The listing builds one solid part. Answer for the finished solid, in the listing's coordinates (mm). A direction names the side the tool comes from. Round coordinates to 2 decimals unless told otherwise and drop trailing zeros. Loops run counter-clockwise (first coordinate to the right, second up) from the corner with the lowest first, then second, coordinate; pieces in that order, holes last. Notation, with made-up numbers: M 23,76.5 L 68,76.5 A15 ccw 68,83.5 Z; hole C 15,87.5 d6. An arc over 180 degrees is marked long. Put each result on its own line as item: value. Start each with the question number.
(1) Section A-A, the plane z = 140 is taken. Determine the outline of the cut face in (x, y), then the cut area to 3 significant figures.
(2) Determine the mould class of faces 5 (the face through (-4.24, 0.751, 137.615)), 6 (the face through (-5, 0, 135)), 7 (the face through (6.466, -2.681, 1.75)) for opening direction Y: released by +Y, released by -Y, zero draft, split by the parting line, or undercut.
(3) Which of the six approach directions +Z, -Z, +X, -X, +Y, -Y give full straight-line access (tool end or side, diameter ignored) to faces 1 (the face through (0, 2, 125)), 2 (the face through (0, 0, -125)), 3 (the face through (5, 0, 135)), 4 (the face through (3.5, 0, 135))?
(4) Flat-ended cylindrical pins translate along their axes: P1, Ø2, axis at y = -4.5, z = 22.5, coming from the -X side; P2, Ø2, axis at y = -0.5, z = 139, coming from the +X side; P3, Ø3.5, axis at y = 0.5, z = 130.5, coming from the -X side; P4, Ø1.2, axis at x = 4.5, z = 136, coming from the -Y side. Find the tip coordinate at first contact, or state that the pin passes through.
(5) Section B-B, the plane z = 19.5 is taken. Determine the outline of the cut face in (x, y).
(6) Straight lines are drawn through the part: line 1 (Z direction, x = 4.3, y = 0); line 2 (Y direction, x = -3.75, z = 140); line 3 (Z direction, x = -0.75, y = 3). For each, find the intervals that lie inside material, in ascending order.
```python
from build123d import *

# Parameters (mm, degrees)
SKETCH1_R                = 7
BOSS_EXTRUDE1_DEPTH      = 125
BOSS_EXTRUDE1_DEPTH_BACK = 125
SKETCH2_W                = 20
SKETCH2_H                = 7
SKETCH2_R                = 2.5
BOSS_EXTRUDE2_DEPTH      = 5
BOSS_EXTRUDE2_DEPTH_BACK = 5
SKETCH4_W                = 7
SKETCH4_H                = 7
CUT_EXTRUDE1_DEPTH       = 20
SKETCH5_R                = 1.5
BOSS_EXTRUDE3_DEPTH      = 5


with BuildPart() as part:
    # Sketch1 → Boss-Extrude1 (new body, two sides)
    with BuildSketch(Plane.XY) as boss_extrude1_sk:
        Circle(SKETCH1_R)
    extrude(amount=BOSS_EXTRUDE1_DEPTH)
    extrude(boss_extrude1_sk.sketch, amount=-BOSS_EXTRUDE1_DEPTH_BACK)

    # Sketch2 → Boss-Extrude2 (add, two sides)
    with BuildSketch(Plane(origin=(0, 0, 0), x_dir=(0, 0, -1), z_dir=(1, 0, 0))) as boss_extrude2_sk:
        with Locations((-135, 0)):
            Rectangle(SKETCH2_W, SKETCH2_H)
        with Locations((-140, 0)):
            Circle(SKETCH2_R, mode=Mode.SUBTRACT)
    extrude(amount=BOSS_EXTRUDE2_DEPTH)
    extrude(boss_extrude2_sk.sketch, amount=-BOSS_EXTRUDE2_DEPTH_BACK)

    # Sketch4 → Cut-Extrude1 (cut)
    with BuildSketch(Plane.XY.offset(145)):
        Rectangle(SKETCH4_W, SKETCH4_H)
    extrude(amount=-CUT_EXTRUDE1_DEPTH, mode=Mode.SUBTRACT)

    # Sketch5 → Boss-Extrude3 (add)
    with BuildSketch(Plane.XY.offset(125)):
        Circle(SKETCH5_R)
    extrude(amount=BOSS_EXTRUDE3_DEPTH)


solid = part.part
```
Recorded:
1. outline: M -5,-3.5 L -3.5,-3.5 L -3.5,-2.5 L -5,-2.5 Z; M -5,2.5 L -3.5,2.5 L -3.5,3.5 L -5,3.5 Z; M 3.5,-3.5 L 5,-3.5 L 5,-2.5 L 3.5,-2.5 Z; M 3.5,2.5 L 5,2.5 L 5,3.5 L 3.5,3.5 Z
1. area: 6.00 mm²
2. face 5: undercut
2. face 6: zero draft
2. face 7: split by the parting line
3. face 1: +Z
3. face 2: -Z, +X, -X, +Y, -Y
3. face 3: +Z, +X, +Y, -Y
3. face 4: +Z, +Y, -Y
4. P1: stops at x = -6.06
4. P2: passes through
4. P3: stops at x = -5
4. P4: stops at y = -3.5
5. outline: C 0,0 d14
6. line 1: z = -125 to 137.5, 142.5 to 145
6. line 2: y = -3.5 to -2.5, 2.5 to 3.5
6. line 3: z = -125 to 125
